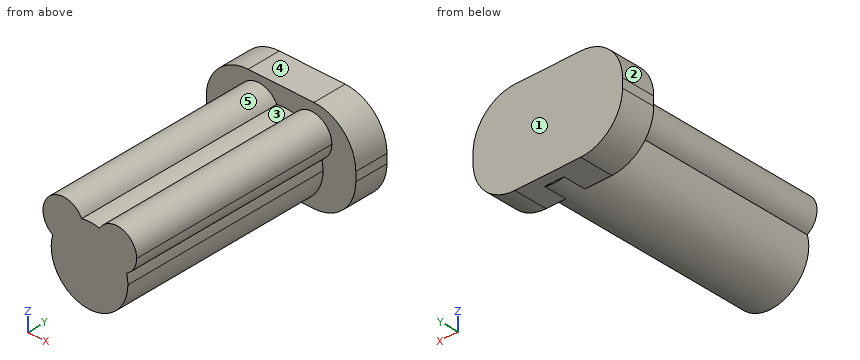
from build123d import *

# Parameters (mm, degrees)
F1_DEPTH      = 57.7
F2_W          = 37.0757319033
F2_H          = 8.3348543849
F3_DEPTH      = 9.1
F3_DEPTH_BACK = 13.9
F4_R          = 10.3811183182


with BuildPart() as f1:
    # F0 (on Front) → F1 (new body)
    with BuildSketch(Plane.XZ):
        with BuildLine():
            ThreePointArc((-8.50842429, -2.055534725), (-0.7108667363, -14.1083254953), (10.1285676568, -4.696719299))
            ThreePointArc((10.1285676568, -4.696719299), (10.0511987024, -3.4863896128), (9.8203512915, -2.2957623088))
            ThreePointArc((9.8203512915, -2.2957623088), (3.867574575, -1.4815476648), (3.107728587, 4.4784129221))
            ThreePointArc((3.107728587, 4.4784129221), (0.8974187737, 4.8049632632), (-1.3280566308, 4.6065600879))
            ThreePointArc((-1.3280566308, 4.6065600879), (-0.9040034744, 3.4731229743), (-0.7599296961, 2.2715641883))
            ThreePointArc((-0.7599296961, 2.2715641883), (-3.3643453928, -2.1658605569), (-8.50842429, -2.055534725))
        make_face()
        with BuildLine():
            ThreePointArc((-1.3280566308, 4.6065600879), (-5.8423978144, 2.2715641883), (-8.50842429, -2.055534725))
            ThreePointArc((-8.50842429, -2.055534725), (-3.3643453928, -2.1658605569), (-0.7599296961, 2.2715641883))
            ThreePointArc((-0.7599296961, 2.2715641883), (-0.9040034744, 3.4731229743), (-1.3280566308, 4.6065600879))
        make_face()
        with BuildLine():
            ThreePointArc((3.107728587, 4.4784129221), (3.867574575, -1.4815476648), (9.8203512915, -2.2957623088))
            ThreePointArc((9.8203512915, -2.2957623088), (7.3750342072, 1.9940419619), (3.107728587, 4.4784129221))
        make_face()
        with BuildLine():
            ThreePointArc((3.107728587, 4.4784129221), (7.3750342072, 1.9940419619), (9.8203512915, -2.2957623088))
            ThreePointArc((9.8203512915, -2.2957623088), (11.6444905303, -0.4866311381), (12.3128471161, 1.9940419619))
            ThreePointArc((12.3128471161, 1.9940419619), (8.6616653793, 6.761281892), (3.107728587, 4.4784129221))
        make_face()
        with BuildLine():
            ThreePointArc((-1.3280566308, 4.6065600879), (-9.2992668658, 5.9973578668), (-8.50842429, -2.055534725))
            ThreePointArc((-8.50842429, -2.055534725), (-5.8423978144, 2.2715641883), (-1.3280566308, 4.6065600879))
        make_face()
    extrude(amount=F1_DEPTH)

    # F2 (on Top) → F3 (join, two sides)
    with BuildSketch(Plane.XY) as f3_sk:
        with Locations((-0.2874098718, -1.4370438876)):
            Rectangle(F2_W, F2_H)
    extrude(amount=F3_DEPTH)
    extrude(f3_sk.sketch, amount=-F3_DEPTH_BACK)

    # F4
    f4_edges = [f1.edges().sort_by_distance(p)[0] for p in [
        (-18.825276, -1.437044, -13.9),
        (-18.825276, -1.437044, 9.1),
        (18.250456, -1.437044, 9.1),
        (18.250456, -1.437044, -13.9),
    ]]
    fillet(f4_edges, radius=F4_R)


solid = f1.part
CAD build for the part. Positions are in the model's coordinates, mm. Face numbers are marked on the shaded views. A direction names the side the tool comes from. Give positions to 0.01 mm unless a question says otherwise; leave off trailing zeros. Order: outer loops, then holes, each group sorted by start corner. A loop starts at its lowest first (then second) coordinate and runs counter-clockwise, first axis right, second up. Notation, with made-up numbers: (12.25, 37.5) - (43.25, 37.5) arc R17 cw to (43.25, 50.5) - close; hole circle Ø8 at (-32, 44). An arc over 180 degrees is marked (long way). Write each question's results on one line, items separated by ' | '.
1. 3-axis set-ups, long thin cutter, end or side, ignore diameter. For the marked faces 4 and 5: which of +Z, -Z, +X, -X, +Y, -Y reach the whole face in a straight line?
Calculated:
face 4: +Z, +X, -X, +Y, -Y | face 5: -Y
2. Saw through at C-C on y = -27. List the corners of the cut face in (x, z).
Calculated:
outline: (-8.51, -2.06) arc R9.51 ccw (long way) to (9.82, -2.3) arc R4.94 ccw (long way) to (3.11, 4.48) arc R9.51 ccw to (-1.33, 4.61) arc R5.08 ccw (long way) to start
3. Saw through at B-B on z = -12.25. List the corners of the cut face in (x, y), and give its area (3 significant figures).
Calculated:
outline: (-14.06, -5.6) - (-5.15, -5.6) - (-5.15, -57.7) - (6.39, -57.7) - (6.39, -5.6) - (13.48, -5.6) - (13.48, 2.73) - (-14.06, 2.73) - close | area: 831 mm2
4. Saw through at D-D on x = 14.5. List the corners of the cut face in (y, z).
Calculated:
outline: (-5.6, -11.51) - (2.73, -11.51) - (2.73, 6.71) - (-5.6, 6.71) - close
5. Pull direction X, two halves, no side cores. Call the marked faces 1, 2 and 3: released by +X, released by -X, zero draft, split by the parting line, or undercut.
Calculated:
face 1: zero draft | face 2: released by -X | face 3: undercut
6. Pin check, flat tips, straight feed: pin 1 (5 mm diameter, centred on x = 10, y = -18, fed in from -Z); pin 2 (12 mm diameter, centred on x = -12, y = -46.5, fed in from -Z); pin 3 (5 mm diameter, centred on y = -23, z = -2, fed in from -X). Stop position of each tip, or through.
Calculated:
pin 1: stops at z = -11.26 | pin 2: stops at z = -11.52 | pin 3: stops at x = -10.61
7. Probe L1, parallel to Y at x = -12, z = -11.5; L2, parallel to X at y = -28.5, z = 5; L3, parallel to X at y = -29, z = -8. List the from-to ranges inside material, lowest first. Write a range as from..to.
Calculated:
L1: y = -5.6..2.73 | L2: x = -10.13..-1.55, 3.46..11.29 | L3: x = -8.29..9.54
8. Saw through at A-A on x = -3. List the corners of the cut face in (y, z), and give its area (3 significant figures).
Calculated:
outline: (-57.7, -13.48) - (-5.6, -13.48) - (-5.6, -13.9) - (2.73, -13.9) - (2.73, 9.1) - (-5.6, 9.1) - (-5.6, 6.48) - (-57.7, 6.48) - close | area: 1,230 mm2
